Geometry: final body of the model. Coordinates: model frame, mm. A direction names the side the tool comes from. Give positions to 0.01 mm unless a question says otherwise; leave off trailing zeros. Loops run counter-clockwise (first coordinate to the right, second up) from the corner with the lowest first, then second, coordinate; pieces in that order, holes last.
from build123d import *

# Parameters (mm, degrees)
F0_W     = 76.2
F0_H     = 50.8
F1_DEPTH = 12.7
F2_W     = 50.8
F2_H     = 50.8
F3_DEPTH = 12.7
F4_W     = 25.4
F4_H     = 19.05
F5_DEPTH = 12.7
F6_W     = 25.4
F6_H     = 50.8
F7_DEPTH = 12.7


with BuildPart() as f1:
    # F0 (on Top) → F1 (new body)
    with BuildSketch(Plane.XY):
        Rectangle(F0_W, F0_H)
    extrude(amount=F1_DEPTH)

    # F2 (on face) → F3 (join)
    with BuildSketch(Plane.XY.offset(12.7)):
        with Locations((12.7, 0)):
            Rectangle(F2_W, F2_H)
    extrude(amount=F3_DEPTH)

    # F4 (on face) → F5 (cut)
    with BuildSketch(Plane.XY.offset(25.4)):
        Rectangle(F4_W, F4_H)
    extrude(amount=-F5_DEPTH, mode=Mode.SUBTRACT)

    # F6 (on face) → F7 (join)
    with BuildSketch(Plane.XY.offset(25.4)):
        with Locations((25.4, 0)):
            Rectangle(F6_W, F6_H)
        Polygon((38.1, -25.4), (38.1, 25.4), (12.7, 25.4), (12.7, 9.525), (12.7, -9.525), (12.7, -25.4), align=None)
    extrude(amount=F7_DEPTH)


solid = f1.part
Item 1: Section query B-B on x = 1.5. Return loops of the section in (y, z) (3 decimals).
Values follow:
outline: (-25.4, 0) - (25.4, 0) - (25.4, 25.4) - (9.525, 25.4) - (9.525, 12.7) - (-9.525, 12.7) - (-9.525, 25.4) - (-25.4, 25.4) - close
Item 2: Pin query (flat end, axial travel): pin 1 (1.5 mm diameter, centred on y = 13.5, z = 30, fed in from -X); pin 2 (5 mm diameter, centred on x = -5.5, y = -14, fed in from +Z); pin 3 (2 mm diameter, centred on y = 14, z = 16, fed in from -X). Return the tip coordinate at first contact, or that it passes through.
Values follow:
pin 1: stops at x = 12.7
pin 2: stops at z = 25.4
pin 3: stops at x = -12.7
Item 3: Set-up query: faces 1 (the face through (-12.7, -18, 19)), 2 (the face through (8, 25.4, 15)), 3 (the face through (0, -9.525, 19)). Return all of +Z, -Z, +X, -X, +Y, -Y with unobstructed straight access to the full face (end or side cutting, diameter ignored); none if empty.
Values follow:
face 1: +Z, -X, +Y, -Y
face 2: +Z, -Z, +X, -X, +Y
face 3: +Z, -X
Item 4: Section query C-C on y = 2. Return loops of the section in (x, z), plus the area to 3 significant figures.
Values follow:
outline: (-38.1, 0) - (38.1, 0) - (38.1, 38.1) - (12.7, 38.1) - (12.7, 12.7) - (-38.1, 12.7) - close
area: 1,610 mm2
Item 5: Section query A-A on z = 16.5. Return loops of the section in (x, y) (3 decimals).
Values follow:
outline: (-12.7, -25.4) - (38.1, -25.4) - (38.1, 25.4) - (-12.7, 25.4) - (-12.7, 9.525) - (12.7, 9.525) - (12.7, -9.525) - (-12.7, -9.525) - close
Item 6: Ray query, probe 1 along Y at (x, z) = (2, 14.5) (3 decimals); probe 2 along Z at (x, y) = (4, 12.5); probe 3 along X at (y, z) = (-17.5, 22). Return the intervals inside material, ascending.
Values follow:
probe 1: y = -25.4 to -9.525, 9.525 to 25.4
probe 2: z = 0 to 25.4
probe 3: x = -12.7 to 38.1
Item 7: Section query D-D on z = 27.5. Return loops of the section in (x, y).
Values follow:
outline: (12.7, -25.4) - (38.1, -25.4) - (38.1, 25.4) - (12.7, 25.4) - close
Item 8: Draft query along Y for faces 4 (the face through (8, -25.4, 15)), 5 (the face through (-19, 0, 12.7)), 6 (the face through (-1, 0, 0)). Return one class per face: +Y half, -Y half, draft (parallel to the pull), parting line (faces both ways), or undercut.
Values follow:
face 4: -Y half
face 5: undercut
face 6: draft
